```python
from build123d import *

# Parameters (mm, degrees)
MODEL_W                 = 3
MODEL_H                 = 3
SALIENTE_EXTRUIR1_DEPTH = 3


with BuildPart() as part:
    # Model → Saliente-Extruir1 (new body)
    with BuildSketch(Plane.XY):
        with BuildLine():
            Line((11.697885884, 299.336573121), (83.697885884, 299.336573121))
            ThreePointArc((83.697885884, 299.336573121), (88.197885884, 294.836573121), (83.697885884, 290.336573121))
            Line((83.697885884, 290.336573121), (11.697885884, 290.336573121))
            ThreePointArc((11.697885884, 290.336573121), (7.197885884, 294.836573121), (11.697885884, 299.336573121))
        make_face()
        with Locations((11.697885884, 294.836573121)):
            Rectangle(MODEL_W, MODEL_H, mode=Mode.SUBTRACT)
        with Locations((20.697885884, 294.836573121)):
            Rectangle(MODEL_W, MODEL_H, mode=Mode.SUBTRACT)
        with Locations((29.697885884, 294.836573121)):
            Rectangle(MODEL_W, MODEL_H, mode=Mode.SUBTRACT)
        with Locations((38.697885884, 294.836573121)):
            Rectangle(MODEL_W, MODEL_H, mode=Mode.SUBTRACT)
        with Locations((47.697885884, 294.836573121)):
            Rectangle(MODEL_W, MODEL_H, mode=Mode.SUBTRACT)
        with Locations((56.697885884, 294.836573121)):
            Rectangle(MODEL_W, MODEL_H, mode=Mode.SUBTRACT)
        with Locations((65.697885884, 294.836573121)):
            Rectangle(MODEL_W, MODEL_H, mode=Mode.SUBTRACT)
        with Locations((74.697885884, 294.836573121)):
            Rectangle(MODEL_W, MODEL_H, mode=Mode.SUBTRACT)
        with Locations((83.697885884, 294.836573121)):
            Rectangle(MODEL_W, MODEL_H, mode=Mode.SUBTRACT)
    extrude(amount=SALIENTE_EXTRUIR1_DEPTH)


solid = part.part
```
Source: CAD feature listing. Evaluate the final solid. Frame: model axes, mm. A direction names the side the tool comes from. Give positions to 0.01 mm unless a question says otherwise; leave off trailing zeros. Write each loop counter-clockwise with the first axis right and the second up, starting at its lowest first coordinate (ties: lowest second). Pieces come first, ordered by that corner, then holes. Notation, with made-up numbers: (-11, 28.5) - (10, 28.5) arc R20 ccw to (10, 51.5) - close; hole circle Ø8 at (59.25, -34.5). An arc over 180 degrees is marked (long way). One line per item, written item: value. Start each with the question number.
Q1. First-contact query: pin 1 Ø1.5 at (y, z) = (298, 1.5) entering from +X. Flat tip, straight axial feed; report the tip coordinate or a pass-through.
Q2. Draft query along Y for faces 1 (the face through (30, 296.337, 1)), 2 (the face through (84, 293.337, 1)), 3 (the face through (47, 299.337, 1)), 4 (the face through (48, 290.337, 1)). Return one class per face: +Y half, -Y half, draft (parallel to the pull), parting line (faces both ways), or undercut.
Q3. Section query D-D, the plane y = 292. Return the cut outline in (x, z), then the cut area to 3 significant figures.
Q4. Section query A-A, the plane x = 38.5. Return the cut outline in (y, z), then the cut area to 3 significant figures.
Q5. Material intervals for probe 1 along Y at (x, z) = (76, 0.1); probe 2 along X at (y, z) = (298.25, 0.1); probe 3 along X at (y, z) = (293, 0.7), sorted ascending. Write a range as from..to.
Q6. Section query B-B, the plane z = 1.7. Count the separate pieces of the cut face and the enclosed holes in it, then the cut area to 3 significant figures.
Q7. Set-up query: faces 5 (the face through (57, 293.337, 1)), 6 (the face through (48, 293, 0)). Return all of +Z, -Z, +X, -X, +Y, -Y with unobstructed straight access to the full face (end or side cutting, diameter ignored); none if empty.
Answer:
1. pin 1: stops at x = 87.5
2. face 1: undercut
2. face 2: undercut
2. face 3: +Y half
2. face 4: -Y half
3. outline: (8.2, 0) - (87.19, 0) - (87.19, 3) - (8.2, 3) - close
3. area: 237 mm2
4. outline: (290.34, 0) - (293.34, 0) - (293.34, 3) - (290.34, 3) - close; (296.34, 0) - (299.34, 0) - (299.34, 3) - (296.34, 3) - close
4. area: 18.0 mm2
5. probe 1: y = 290.34..293.34, 296.34..299.34
5. probe 2: x = 8.77..86.63
5. probe 3: x = 7.59..87.81
6. separate pieces: 1
6. enclosed holes: 9
6. area: 631 mm2
7. face 5: +Z, -Z
7. face 6: -Z, +X, -X, +Y, -Y
